Check sheet for the drawn part. Datum: minimum x, y, z corner. Units: mm. Give positions to 0.01 mm unless a question says otherwise; leave off trailing zeros. Order: outer loops, then holes, each group sorted by start corner. A loop starts at its lowest first (then second) coordinate and runs counter-clockwise, first axis right, second up.
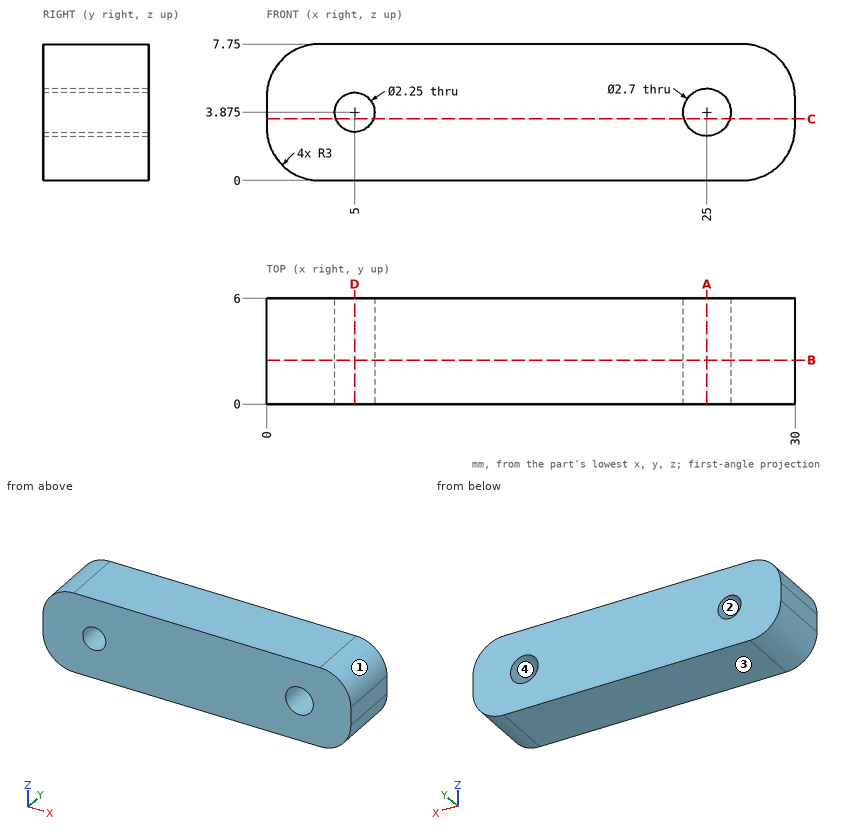
Item 1: Draft check along X on the marked faces 1, 2, 3 and 4. Enter one of: released by +X, released by -X, zero draft, split by the parting line, or undercut.
Reported:
face 1: released by +X
face 2: undercut
face 3: zero draft
face 4: undercut
Item 2: Sectioned sample at B-B (y = 2.5). Enter the section's corners in (x, z) (3 decimals).
Reported:
outline: (0, 3) arc R3 ccw to (3, 0) - (27, 0) arc R3 ccw to (30, 3) - (30, 4.75) arc R3 ccw to (27, 7.75) - (3, 7.75) arc R3 ccw to (0, 4.75) - close; hole circle Ø2.25 at (5, 3.875); hole circle Ø2.7 at (25, 3.875)
Item 3: Gauge pin test, flat end, axial feed: pin 1 (1.6 mm diameter, centred on x = 25, z = 3.875, fed in from +Y) (1 decimal). Record the tip position at first contact, or that the pin passes through.
Reported:
pin 1: passes through
Item 4: Sectioned sample at D-D (x = 5). Enter the section's corners in (y, z).
Reported:
outline: (0, 0) - (6, 0) - (6, 2.75) - (0, 2.75) - close; (0, 5) - (6, 5) - (6, 7.75) - (0, 7.75) - close
Item 5: Sectioned sample at A-A (x = 25). Enter the section's corners in (y, z) (3 decimals).
Reported:
outline: (0, 0) - (6, 0) - (6, 2.525) - (0, 2.525) - close; (0, 5.225) - (6, 5.225) - (6, 7.75) - (0, 7.75) - close
Item 6: Scan lines: L1, parallel to X at y = 0.95, z = 3.75; L2, parallel to Z at x = 25, y = 2 (3 decimals); L3, parallel to X at y = 3.7, z = 3.25. Record each from-to range of solid material in increasing order.
Reported:
L1: x = 0 to 3.88, 6.12 to 23.66, 26.34 to 30
L2: z = 0 to 2.525, 5.225 to 7.75
L3: x = 0 to 4.06, 5.94 to 23.8, 26.2 to 30
Item 7: Sectioned sample at C-C (z = 3.5). Enter the section's corners in (x, y), and give its area (3 significant figures).
Reported:
outline: (0, 0) - (3.94, 0) - (3.94, 6) - (0, 6) - close; (6.06, 0) - (23.7, 0) - (23.7, 6) - (6.06, 6) - close; (26.3, 0) - (30, 0) - (30, 6) - (26.3, 6) - close
area: 152 mm2
